Part model, mm, in its own coordinate system. Face numbers are marked on the shaded views. Coordinates: 2 decimals unless noted, no trailing zeros. Loops run counter-clockwise (first coordinate to the right, second up) from the corner with the lowest first, then second, coordinate; pieces in that order, holes last. Notation, with made-up numbers: (83, 32) - (103, 32) arc R15 cw to (103, 55) - close; hole circle Ø6 at (84.5, 41). An arc over 180 degrees is marked (long way). Answer as CSV lines item,"result".
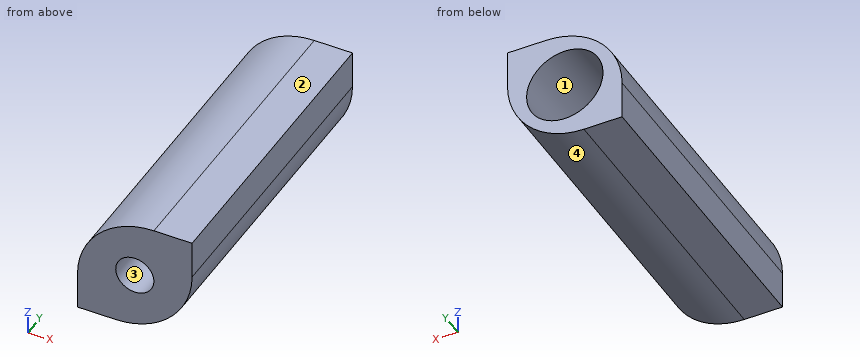
from build123d import *

# Parameters (mm, degrees)
SKETCH_1_R            = 6
EXTRUDE_1_DEPTH       = 40
SKETCH_2_R            = 5
CUT_EXTRUDE_2_DEPTH   = 30
SKETCH_3_R            = 2.5
CUT_EXTRUDE_4_DEPTH   = 10
SKETCH_5_R            = 16
SKETCH_5_R_2          = 6
EXTRUDE_1_2_DEPTH     = 40
SKETCH_6_W            = 32
SKETCH_6_H            = 32
SKETCH_6_W_2          = 12
SKETCH_6_H_2          = 12
EXTRUDE_2_DEPTH       = 40
SKETCH_7_W            = 35
SKETCH_7_H            = 35
SKETCH_7_W_2          = 15
SKETCH_7_H_2          = 15
CUT_EXTRUDE_2_2_DEPTH = 46.956501172
FILLET_1_R            = 10


with BuildPart() as part:
    # 草圖1 → Extrude 1 (new body)
    with BuildSketch(Plane(origin=(0, 0, 0), x_dir=(1, 0, 0), z_dir=(0, 1, 0))):
        with Locations(Location((0, 0, 0), (0, 0, 270))):
            Circle(SKETCH_1_R)
    extrude(amount=EXTRUDE_1_DEPTH)

    # 草圖2 → Cut-Extrude 2 (cut)
    with BuildSketch(Plane(origin=(0, 40, 0), x_dir=(1, 0, 0), z_dir=(0, 1, 0))):
        with Locations(Location((0, 0, 0), (0, 0, 270))):
            Circle(SKETCH_2_R)
    extrude(amount=-CUT_EXTRUDE_2_DEPTH, mode=Mode.SUBTRACT)

    # 草圖3 → 除料-伸長4 (cut)
    with BuildSketch(Plane.XZ):
        with Locations(Location((0, 0, 0), (0, 0, 270))):
            Circle(SKETCH_3_R)
    extrude(amount=-CUT_EXTRUDE_4_DEPTH, mode=Mode.SUBTRACT)

    # 草圖5 → Extrude 1 2 (add)
    with BuildSketch(Plane(origin=(0, 0, 0), x_dir=(1, 0, 0), z_dir=(0, 1, 0))):
        Circle(SKETCH_5_R)
        Circle(SKETCH_5_R_2, mode=Mode.SUBTRACT)
    extrude(amount=EXTRUDE_1_2_DEPTH)

    # 草圖6 → 伸長-薄件2 (add)
    with BuildSketch(Plane(origin=(0, 40, 0), x_dir=(1, 0, 0), z_dir=(0, 1, 0))):
        Rectangle(SKETCH_6_W, SKETCH_6_H)
        Rectangle(SKETCH_6_W_2, SKETCH_6_H_2, mode=Mode.SUBTRACT)
    extrude(amount=-EXTRUDE_2_DEPTH)

    # 草圖7 → Cut-Extrude 2 2 (cut, through all)
    with BuildSketch(Plane(origin=(0, 40, 0), x_dir=(1, 0, 0), z_dir=(0, 1, 0))):
        Rectangle(SKETCH_7_W, SKETCH_7_H)
        Rectangle(SKETCH_7_W_2, SKETCH_7_H_2, mode=Mode.SUBTRACT)
    extrude(amount=-CUT_EXTRUDE_2_2_DEPTH, mode=Mode.SUBTRACT)

    # 圓角1
    fillet_1_edges = [part.edges().sort_by_distance(p)[0] for p in [
        (-7.5, 20, 7.5),
        (7.5, 20, -7.5),
    ]]
    fillet(fillet_1_edges, radius=FILLET_1_R)


solid = part.part
Q1. Saw through at A-A (y = 7.5). Give the cut face in (x, z).
Results:
outline,"(-7.5, -7.5) - (-2.5, -7.5) arc R10 ccw to (7.5, 2.5) - (7.5, 7.5) - (2.5, 7.5) arc R10 ccw to (-7.5, -2.5) - close; hole circle Ø5 at (0, 0)"
Q2. Saw through at C-C (z = 0). Give the cut face in (x, y).
Results:
outline,"(-7.18, 0) - (-2.5, 0) - (-2.5, 10) - (-5, 10) - (-5, 40) - (-7.18, 40) - close; (2.5, 0) - (7.18, 0) - (7.18, 40) - (5, 40) - (5, 10) - (2.5, 10) - close"
Q3. Flat gauge pins, fed straight in: pin 1 (6 mm diameter, centred on x = 0, z = 0, fed in from +Y); pin 2 (5 mm diameter, centred on x = -3.5, y = 21, fed in from +Z); pin 3 (5 mm diameter, centred on y = 22.5, z = -5, fed in from +X). Where does each tip first touch, or does it go through?
Results:
pin 1,"stops at y = 10"
pin 2,"stops at z = 6.87"
pin 3,"stops at x = 6.16"
Q4. Saw through at B-B (x = 0). Give the cut face in (y, z), then the cut area to 3 significant figures.
Results:
outline,"(0, -7.18) - (40, -7.18) - (40, -5) - (10, -5) - (10, -2.5) - (0, -2.5) - close; (0, 2.5) - (10, 2.5) - (10, 5) - (40, 5) - (40, 7.18) - (0, 7.18) - close"
area,"225 mm^2"
Q5. Two-plate mould, pull along Z, no slides. Class the marked faces 1, 2, 3 and 4: released by +Z, released by -Z, zero draft, split by the parting line, or undercut.
Results:
face 1,"undercut"
face 2,"released by +Z"
face 3,"undercut"
face 4,"released by -Z"
Q6. Wall check: L1, parallel to Y at x = 1.5, z = 4.5; L2, parallel to Z at x = 0.25, y = 34; L3, parallel to X at y = 17, z = 0. Give the ranges that are in metal, low to high.
Results:
L1,"y = 0 to 10"
L2,"z = -7.11 to -4.99, 4.99 to 7.24"
L3,"x = -7.18 to -5, 5 to 7.18"
Q7. Saw through at D-D (y = 28.5). Give the cut face in (x, z).
Results:
outline,"(-7.5, -7.5) - (-2.5, -7.5) arc R10 ccw to (7.5, 2.5) - (7.5, 7.5) - (2.5, 7.5) arc R10 ccw to (-7.5, -2.5) - close; hole circle Ø10 at (0, 0)"
